Could you check a few things on this model? Use its own coordinates, in mm. Coordinates: 2 decimals unless noted, no trailing zeros. Write each loop counter-clockwise with the first axis right and the second up, starting at its lowest first coordinate (ties: lowest second). Pieces come first, ordered by that corner, then holes. Notation, with made-up numbers: M 75,-31.75 L 110,-31.75 A26 cw 110,-5.75 Z; hole C 34.5,8 d7. An arc over 180 degrees is marked long. Write item = value, one per line.
```python
from build123d import *

# Parameters (mm, degrees)
F0_R     = 200
F1_DEPTH = 3
F2_D     = 5
F2_DEPTH = 60
F2_TIP   = 1.5021515476
F3_R     = 1
F4_D     = 80
F4_DEPTH = 60
F4_TIP   = 24.0344247611


with BuildPart() as f1:
    # F0 (on Front) → F1 (new body)
    with BuildSketch(Plane.XZ):
        Circle(F0_R)
    extrude(amount=F1_DEPTH)

    # F2
    with Locations(Plane(origin=(0, 0, 0), x_dir=(1, 0, 0), z_dir=(0, 1, 0))):
        with Locations((-15, -186.6666666667), (15, -186.6666666667)):
            Hole(F2_D / 2, depth=F2_DEPTH)
            with Locations((0, 0, -(F2_DEPTH + F2_TIP / 2))):  # 118° drill point
                Cone(0, F2_D / 2, F2_TIP, mode=Mode.SUBTRACT)

    # F3
    f3_edges = [f1.edges().sort_by_distance(p)[0] for p in [
        (-200, -3, 0),
        (-200, 0, 0),
    ]]
    fillet(f3_edges, radius=F3_R)

    # F4
    with Locations(Plane(origin=(0, 0, 0), x_dir=(1, 0, 0), z_dir=(0, 1, 0))):
        with Locations((0, 0)):
            Hole(F4_D / 2, depth=F4_DEPTH)
            with Locations((0, 0, -(F4_DEPTH + F4_TIP / 2))):  # 118° drill point
                Cone(0, F4_D / 2, F4_TIP, mode=Mode.SUBTRACT)


solid = f1.part
```
Item 1: If we mould it in two halves opening along Z, with no side actions, what happens to faces 1 (the face through (-3, 0, -41)), 2 (the face through (190.764, -1.493, 60.075)), 3 (the face through (8.67, -1.52, 39.05))? For each: pulls with the +Z half, pulls with the -Z half, needs draft (parallel to the pull), parting line crosses it, or undercut.
Numbers:
face_1 = needs draft
face_2 = parting line crosses it
face_3 = undercut
Item 2: I'm going to push flat-ended pins straight in: P1, Ø1.5, axis at y = -2.5, z = 107.5, coming from the +X side; P2, Ø3, axis at x = 64, z = -139, coming from the +Y side. Where does each tip first touch, or does it pass through?
Numbers:
P1 = 169.07
P2 = 0
Item 3: If I drill on line 1 along Z through (x, y) = (-15, -1.75); line 2 along Z through (x, y) = (0, -1.8); line 3 along Z through (x, y) = (0, -0.75), over which ranges is the centre line in solid material (lowest first)?
Numbers:
line_1 = -199.44 to -37.08, 37.08 to 184.17, 189.17 to 199.44
line_2 = -200 to -40, 40 to 200
line_3 = -199.97 to -40, 40 to 199.97
Item 4: Imagine slicing it at B-B (z = 0). Write out the boundary of the cut face in (x, y).
Numbers:
outline = M -200,-2 A1 ccw -199,-3 L -40,-3 L -40,0 L -199,0 A1 ccw -200,-1 Z; M 40,-3 L 199,-3 A1 ccw 200,-2 L 200,-1 A1 ccw 199,0 L 40,0 Z
Item 5: Imagine slicing it at A-A (x = 0). Write out the boundary of the cut face in (y, z), and give its area (3 significant figures).
Numbers:
outline = M -3,-199 A1 ccw -2,-200 L -1,-200 A1 ccw 0,-199 L 0,-40 L -3,-40 Z; M -3,40 L 0,40 L 0,199 A1 ccw -1,200 L -2,200 A1 ccw -3,199 Z
area = 959 mm²
